from build123d import *

# Parameters (mm, degrees)
SKETCH_1_R          = 1.8
SKETCH_1_R_2        = 1.55
EXTRUDE_1_DEPTH     = 4
SKETCH_3_R          = 2.5
CUT_EXTRUDE_2_DEPTH = 10
FILLET_1_R          = 1


with BuildPart() as part:
    # 草图1 → 凸台-拉伸1 (new body)
    with BuildSketch(Plane.XY):
        with BuildLine():
            Line((35, 46.920144927), (-35, 46.920144927))
            Line((-35, 46.920144927), (-35, 32.810744327))
            Line((-35, 32.810744327), (-27, 28.191942173))
            Line((-27, 28.191942173), (-27, 23.009508904))
            ThreePointArc((-27, 23.009508904), (-16.614935725, -4.665079356), (-35, -27.810744327))
            Line((-35, -27.810744327), (-35, -46.920144927))
            Line((-35, -46.920144927), (-35, -49.920144927))
            Line((-35, -49.920144927), (35, -49.920144927))
            Line((35, -49.920144927), (35, -46.920144927))
            Line((35, -46.920144927), (35, -27.810744327))
            ThreePointArc((35, -27.810744327), (16.334866743, -2.254950607), (30.958156738, 25.81006644))
            Line((30.958156738, 25.81006644), (35, 32.810744327))
            Line((35, 32.810744327), (35, 46.920144927))
        make_face()
        with Locations((-16.1979618, -30.0520382)):
            Circle(SKETCH_1_R, mode=Mode.SUBTRACT)
        with Locations((16.1979618, -30.0520382)):
            Circle(SKETCH_1_R, mode=Mode.SUBTRACT)
        with Locations((-3.75, 0)):
            Circle(SKETCH_1_R, mode=Mode.SUBTRACT)
        with Locations((-16.1979618, 30.0520382)):
            Circle(SKETCH_1_R, mode=Mode.SUBTRACT)
        with Locations((-3.05, 40)):
            Circle(SKETCH_1_R_2, mode=Mode.SUBTRACT)
        with Locations((3.75, 0)):
            Circle(SKETCH_1_R, mode=Mode.SUBTRACT)
        with Locations((16.1979618, 30.0520382)):
            Circle(SKETCH_1_R, mode=Mode.SUBTRACT)
        with Locations((11.95, 40)):
            Circle(SKETCH_1_R_2, mode=Mode.SUBTRACT)
    extrude(amount=EXTRUDE_1_DEPTH)

    # 草图3 → 切除-拉伸2 (cut)
    with BuildSketch(Plane(origin=(0, 0, 0), x_dir=(-1, 0, 0), z_dir=(0, 0, -1))):
        with Locations((-15, 20)):
            Circle(SKETCH_3_R)
        with Locations((15, 20)):
            Circle(SKETCH_3_R)
        with Locations((15, -20)):
            Circle(SKETCH_3_R)
        with Locations((-15, -20)):
            Circle(SKETCH_3_R)
    extrude(amount=-CUT_EXTRUDE_2_DEPTH, mode=Mode.SUBTRACT)

    # 圆角1
    fillet_1_edges = [part.edges().sort_by_distance(p)[0] for p in [
        (35, -27.810744327, 2),
        (35, -49.920144927, 2),
        (-35, -49.920144927, 2),
        (-35, -27.810744327, 2),
        (-27, 23.009508904, 2),
        (-27, 28.191942173, 2),
        (-35, 32.810744327, 2),
        (-35, 46.920144927, 2),
        (35, 46.920144927, 2),
        (35, 32.810744327, 2),
        (30.958156738, 25.81006644, 2),
    ]]
    fillet(fillet_1_edges, radius=FILLET_1_R)


solid = part.part
The listing builds one solid part. Answer for the finished solid, in the listing's coordinates (mm). A direction names the side the tool comes from. Coordinates: 2 decimals unless noted, no trailing zeros. Loops run counter-clockwise (first coordinate to the right, second up) from the corner with the lowest first, then second, coordinate; pieces in that order, holes last. Notation, with made-up numbers: M 88.5,-26 L 94.5,-26 A22 cw 94.5,-1 Z; hole C 89.25,-22.5 d6. An arc over 180 degrees is marked long. Answer in a Markdown table with one row per item.
1) Find the intervals of material crossed by probe 1 along X at (y, z) = (-29, 1.25); probe 2 along Y at (x, z) = (13, 0.85); probe 3 along Y at (x, z) = (-3.05, 2.1), in increasing order.
Answers below:
| item | result |
|---|---|
| probe 1 | -35 to -17.66, -14.74 to 14.74, 17.66 to 35 |
| probe 2 | -49.92 to -21.5, -18.5 to 18.5, 21.5 to 38.86, 41.14 to 46.92 |
| probe 3 | -49.92 to -1.66, 1.66 to 38.45, 41.55 to 46.92 |
2) Determine the mould class of faces 3 (the cylindrical face through (-2.033, 0.541, 1.972)), 4 (the flat face through (0, -1, 4)), 5 (the flat face through (0, -49.92, 2)) for opening direction Y: released by +Y, released by -Y, zero draft, split by the parting line, or undercut.
Answers below:
| item | result |
|---|---|
| face 3 | undercut |
| face 4 | zero draft |
| face 5 | released by -Y |
3) Find section D-D (x = -21.5). Determine the outline of the cut face in (y, z), then the cut area to 3 significant figures.
Answers below:
| item | result |
|---|---|
| outline | M -49.92,0 L -16.95,0 L -16.95,4 L -49.92,4 Z; M 16.95,0 L 46.92,0 L 46.92,4 L 16.95,4 Z |
| area | 252 mm^2 |
4) Find section C-C (x = -3.05). Determine the outline of the cut face in (y, z).
Answers below:
| item | result |
|---|---|
| outline | M -49.92,0 L -1.66,0 L -1.66,4 L -49.92,4 Z; M 1.66,0 L 38.45,0 L 38.45,4 L 1.66,4 Z; M 41.55,0 L 46.92,0 L 46.92,4 L 41.55,4 Z |
5) Which of the six approach directions +Z, -Z, +X, -X, +Y, -Y give full straight-line access (tool end or side, diameter ignored) to faces 1 (the flat face through (-31, 30.5, 2)), 2 (the cylindrical face through (-3.386, 38.487, 1.972))?
Answers below:
| item | result |
|---|---|
| face 1 | +Z, -Z, -X |
| face 2 | +Z, -Z |
6) Find section B-B (z = 0.6). Count the separate pieces of the cut face and the enclosed holes in it, then the cut area to 3 significant figures.
Answers below:
| item | result |
|---|---|
| separate pieces | 1 |
| enclosed holes | 12 |
| area | 5,060 mm^2 |
7) Given pin 1 (3 mm diameter, centred on x = 15, y = 20, fed in from -Z); pin 2 (1.2 mm diameter, centred on y = 24.5, z = 1.5, fed in from -X); pin 3 (1 mm diameter, centred on y = -21, z = 2, fed in from +X), each flat-ended and moving along its own axis, determine where each tip first touches the part or whether it passes through.
Answers below:
| item | result |
|---|---|
| pin 1 | through |
| pin 2 | x = -27 |
| pin 3 | x = 25.33 |
8) Find section A-A (y = 20). Determine the outline of the cut face in (x, z).
Answers below:
| item | result |
|---|---|
| outline | M -23.89,0 L -17.5,0 L -17.5,4 L -23.89,4 Z; M -12.5,0 L 12.5,0 L 12.5,4 L -12.5,4 Z; M 17.5,0 L 23.89,0 L 23.89,4 L 17.5,4 Z |
